Geometry check sheet. Reference: the model listing, model coordinates, mm. A direction names the side the tool comes from. Give positions to 0.01 mm unless a question says otherwise; leave off trailing zeros. Order: outer loops, then holes, each group sorted by start corner. A loop starts at its lowest first (then second) coordinate and runs counter-clockwise, first axis right, second up.
from build123d import *

# Parameters (mm, degrees)
EXTRUDE_1_DEPTH     = 30
CHAMFER_1_SIZE      = 10
CHAMFER_2_SIZE      = 5
SKETCH_2_R          = 30
EXTRUDE_2_DEPTH     = 41
EXTRUDE_3_DEPTH     = 10
SKETCH_4_R          = 25
EXTRUDE_4_DEPTH     = 3
SKETCH_5_R          = 7
EXTRUDE_5_DEPTH     = 35
CUT_EXTRUDE_1_REACH = 147.399
SKETCH_6_R          = 2.75
SKETCH_8_R          = 25
CUT_EXTRUDE_2_DEPTH = 5
SKETCH_9_R          = 7
CUT_EXTRUDE_3_DEPTH = 31.5
EXTRUDE_6_DEPTH     = 9
CHAMFER_3_SIZE      = 0.5
SKETCH_11_R         = 2
CUT_EXTRUDE_4_DEPTH = 30
SKETCH_12_R         = 2.5
CUT_EXTRUDE_5_DEPTH = 30
CHAMFER_4_SIZE      = 1


with BuildPart() as part:
    # 草图1 → 凸台-拉伸1 (new, symmetric)
    with BuildSketch(Plane(origin=(0, 0, 0), x_dir=(0, 0, -1), z_dir=(1, 0, 0))):
        Polygon((0, 0), (0, -40.5), (60, -40.5), (60, 40), (40, 60), (-28, 60), (-28, 0), align=None)
    extrude(amount=EXTRUDE_1_DEPTH, both=True)

    # 倒角1
    chamfer_1_edges = [part.edges().sort_by_distance(p)[0] for p in [
        (0, 0, 0),
    ]]
    chamfer(chamfer_1_edges, length=CHAMFER_1_SIZE)

    # 倒角2
    chamfer_2_edges = [part.edges().sort_by_distance(p)[0] for p in [
        (-30, 0, 19),
        (30, -0.25, -60),
        (30, 50, -50),
        (-30, -25.25, 0),
        (30, -25.25, 0),
        (-30, -5, 5),
        (30, -5, 5),
        (30, 60, -6),
        (30, 0, 19),
        (-30, 60, -6),
        (-30, 50, -50),
        (-30, -0.25, -60),
    ]]
    chamfer(chamfer_2_edges, length=CHAMFER_2_SIZE)

    # 草图2 → 凸台-拉伸2 (add)
    with BuildSketch(Plane.XY.offset(28)):
        with Locations((0, 30)):
            Circle(SKETCH_2_R)
    extrude(amount=EXTRUDE_2_DEPTH)

    # 草图3 → 凸台-拉伸3 (add)
    with BuildSketch(Plane.XY.offset(69)):
        Polygon((-30, 30), (-30, 5), (-25, 0), (25, 0), (30, 5), (30, 30), (30, 55), (25, 60), (0, 60), (-25, 60), (-30, 55), align=None)
    extrude(amount=-EXTRUDE_3_DEPTH)

    # 草图4 → 凸台-拉伸4 (add)
    with BuildSketch(Plane.XY.offset(69)):
        with Locations((0, 30)):
            Circle(SKETCH_4_R)
    extrude(amount=EXTRUDE_4_DEPTH)

    # 草图5 → 凸台-拉伸5 (add)
    with BuildSketch(Plane.XY.offset(69)):
        with Locations((0, 30)):
            Circle(SKETCH_5_R)
    extrude(amount=EXTRUDE_5_DEPTH)

    # 草图6 → 切除-拉伸1 (cut, up to next)
    with BuildSketch(Plane.XY.offset(69), mode=Mode.PRIVATE) as cut_extrude_1_sk1:
        with Locations((-24.748737342, 54.748737342)):
            Circle(SKETCH_6_R)
    cut_extrude_1_tool1 = extrude(cut_extrude_1_sk1.sketch, amount=-CUT_EXTRUDE_1_REACH, mode=Mode.PRIVATE) & part.part
    # 草图6 → 切除-拉伸1 (cut, up to next)
    with BuildSketch(Plane.XY.offset(69), mode=Mode.PRIVATE) as cut_extrude_1_sk2:
        with Locations((24.748737342, 54.748737342)):
            Circle(SKETCH_6_R)
    cut_extrude_1_tool2 = extrude(cut_extrude_1_sk2.sketch, amount=-CUT_EXTRUDE_1_REACH, mode=Mode.PRIVATE) & part.part
    # 草图6 → 切除-拉伸1 (cut, up to next)
    with BuildSketch(Plane.XY.offset(69), mode=Mode.PRIVATE) as cut_extrude_1_sk3:
        with Locations((24.748737342, 5.251262658)):
            Circle(SKETCH_6_R)
    cut_extrude_1_tool3 = extrude(cut_extrude_1_sk3.sketch, amount=-CUT_EXTRUDE_1_REACH, mode=Mode.PRIVATE) & part.part
    # 草图6 → 切除-拉伸1 (cut, up to next)
    with BuildSketch(Plane.XY.offset(69), mode=Mode.PRIVATE) as cut_extrude_1_sk4:
        with Locations((-24.748737342, 5.251262658)):
            Circle(SKETCH_6_R)
    cut_extrude_1_tool4 = extrude(cut_extrude_1_sk4.sketch, amount=-CUT_EXTRUDE_1_REACH, mode=Mode.PRIVATE) & part.part
    add(cut_extrude_1_tool1.solids().sort_by_distance((-24.748737, 54.748737, 69))[0], mode=Mode.SUBTRACT)
    add(cut_extrude_1_tool2.solids().sort_by_distance((24.748737, 54.748737, 69))[0], mode=Mode.SUBTRACT)
    add(cut_extrude_1_tool3.solids().sort_by_distance((24.748737, 5.251263, 69))[0], mode=Mode.SUBTRACT)
    add(cut_extrude_1_tool4.solids().sort_by_distance((-24.748737, 5.251263, 69))[0], mode=Mode.SUBTRACT)

    # 草图8 → 切除-拉伸2 (cut)
    with BuildSketch(Plane.XZ.offset(40.5)):
        with Locations(Location((0, -30, 0), (0, 0, 270))):
            Circle(SKETCH_8_R)
    extrude(amount=-CUT_EXTRUDE_2_DEPTH, mode=Mode.SUBTRACT)

    # 草图9 → 切除-拉伸3 (cut)
    with BuildSketch(Plane.XZ.offset(40.5)):
        with Locations(Location((0, -30, 0), (0, 0, 270))):
            Circle(SKETCH_9_R)
    extrude(amount=-CUT_EXTRUDE_3_DEPTH, mode=Mode.SUBTRACT)

    # 草图10 → 凸台-拉伸6 (add)
    with BuildSketch(Plane(origin=(0, 0, 0), x_dir=(0, 0, -1), z_dir=(1, 0, 0))):
        with BuildLine():
            Line((-98.5, 32.5), (-83.5, 32.5))
            ThreePointArc((-83.5, 32.5), (-81, 30), (-83.5, 27.5))
            Line((-83.5, 27.5), (-98.5, 27.5))
            ThreePointArc((-98.5, 27.5), (-101, 30), (-98.5, 32.5))
        make_face()
    extrude(amount=EXTRUDE_6_DEPTH)

    # 倒角3
    chamfer_3_edges = [part.edges().sort_by_distance(p)[0] for p in [
        (9, 30, 101),
        (9, 27.5, 91),
        (9, 30, 81),
        (9, 32.5, 91),
    ]]
    chamfer(chamfer_3_edges, length=CHAMFER_3_SIZE)

    # 草图11 → 切除-拉伸4 (cut)
    with BuildSketch(Plane.XZ.offset(40.5)):
        with Locations(Location((-24.748737342, -5.251262658, 0), (0, 0, 270))):
            Circle(SKETCH_11_R)
        with Locations(Location((24.748737342, -5.251262658, 0), (0, 0, 270))):
            Circle(SKETCH_11_R)
        with Locations(Location((24.748737342, -54.748737342, 0), (0, 0, 270))):
            Circle(SKETCH_11_R)
        with Locations(Location((-24.748737342, -54.748737342, 0), (0, 0, 270))):
            Circle(SKETCH_11_R)
    extrude(amount=-CUT_EXTRUDE_4_DEPTH, mode=Mode.SUBTRACT)

    # 草图12 → 切除-拉伸5 (cut)
    with BuildSketch(Plane.XY.offset(104)):
        with Locations((0, 30)):
            Circle(SKETCH_12_R)
    extrude(amount=-CUT_EXTRUDE_5_DEPTH, mode=Mode.SUBTRACT)

    # 倒角4
    chamfer_4_edges = [part.edges().sort_by_distance(p)[0] for p in [
        (-7, 30, 104),
    ]]
    chamfer(chamfer_4_edges, length=CHAMFER_4_SIZE)


solid = part.part
Item 1: Set-up check for faces 4 (the flat face through (0, -9, -30)), 5 (the flat face through (0, 0, 64)), 6 (the cylindrical face through (-25.107, 57.475, 64.07)): record each of +Z, -Z, +X, -X, +Y, -Y from which the full face is reachable in a straight line by a thin tool's end or side.
Reported:
face 4: -Y
face 5: +Z, +X, -X, -Y
face 6: +Z
Item 2: Sectioned sample at A-A (z = 17.5). Enter the section's corners in (x, y).
Reported:
outline: (-30, 5) - (-25, 0) - (25, 0) - (30, 5) - (30, 55) - (25, 60) - (-25, 60) - (-30, 55) - close
Item 3: Sectioned sample at D-D (x = 20). Enter the section's corners in (y, z).
Reported:
outline: (-40.5, -60) - (40, -60) - (60, -40) - (60, 28) - (52.36, 28) - (52.36, 59) - (60, 59) - (60, 69) - (45, 69) - (45, 72) - (15, 72) - (15, 69) - (0, 69) - (0, 59) - (7.64, 59) - (7.64, 28) - (0, 28) - (0, 10) - (-10, 0) - (-40.5, 0) - (-40.5, -15) - (-35.5, -15) - (-35.5, -45) - (-40.5, -45) - close
Item 4: Sectioned sample at B-B (y = -17). Enter the section's corners in (x, z).
Reported:
outline: (-30, -55) - (-25, -60) - (25, -60) - (30, -55) - (30, -5) - (25, 0) - (-25, 0) - (-30, -5) - close; hole circle Ø4 at (-24.75, -54.75); hole circle Ø4 at (-24.75, -5.25); hole circle Ø14 at (0, -30); hole circle Ø4 at (24.75, -54.75); hole circle Ø4 at (24.75, -5.25)
Item 5: Gauge pin test, flat ends, axial feed: pin 1 (12 mm diameter, centred on x = -17.5, z = 36, fed in from +Y); pin 2 (5.5 mm diameter, centred on x = -3.5, z = 19, fed in from -Y); pin 3 (6 mm diameter, centred on x = 11.5, z = 10, fed in from -Y). Record the tip position at first contact, or that the pin passes through.
Reported:
pin 1: stops at y = 57.71
pin 2: stops at y = 0
pin 3: stops at y = -3
Item 6: Draft check along X on faces 1 (the flat face through (0, 27, 104)), 2 (the cylindrical face through (24.84, -25.71, -52.75)), 3 (the flat face through (28, -24, -3)). Enter one of: released by +X, released by -X, zero draft, split by the parting line, or undercut.
Reported:
face 1: zero draft
face 2: undercut
face 3: released by +X
Item 7: Sectioned sample at C-C (y = 21). Enter the section's corners in (x, z).
Reported:
outline: (-30, -55) - (-25, -60) - (25, -60) - (30, -55) - (30, 28) - (28.62, 28) - (28.62, 59) - (30, 59) - (30, 69) - (23.32, 69) - (23.32, 72) - (-23.32, 72) - (-23.32, 69) - (-30, 69) - (-30, 59) - (-28.62, 59) - (-28.62, 28) - (-30, 28) - close
Item 8: Scan lines: L1, parallel to Z at x = 22.5, y = 17; L2, parallel to Z at x = 6.5, y = -3; L3, parallel to Y at x = -11, z = -36. Record each from-to range of solid material in increasing order.
Reported:
L1: z = -60 to 69
L2: z = -60 to 7
L3: y = -35.5 to 60
